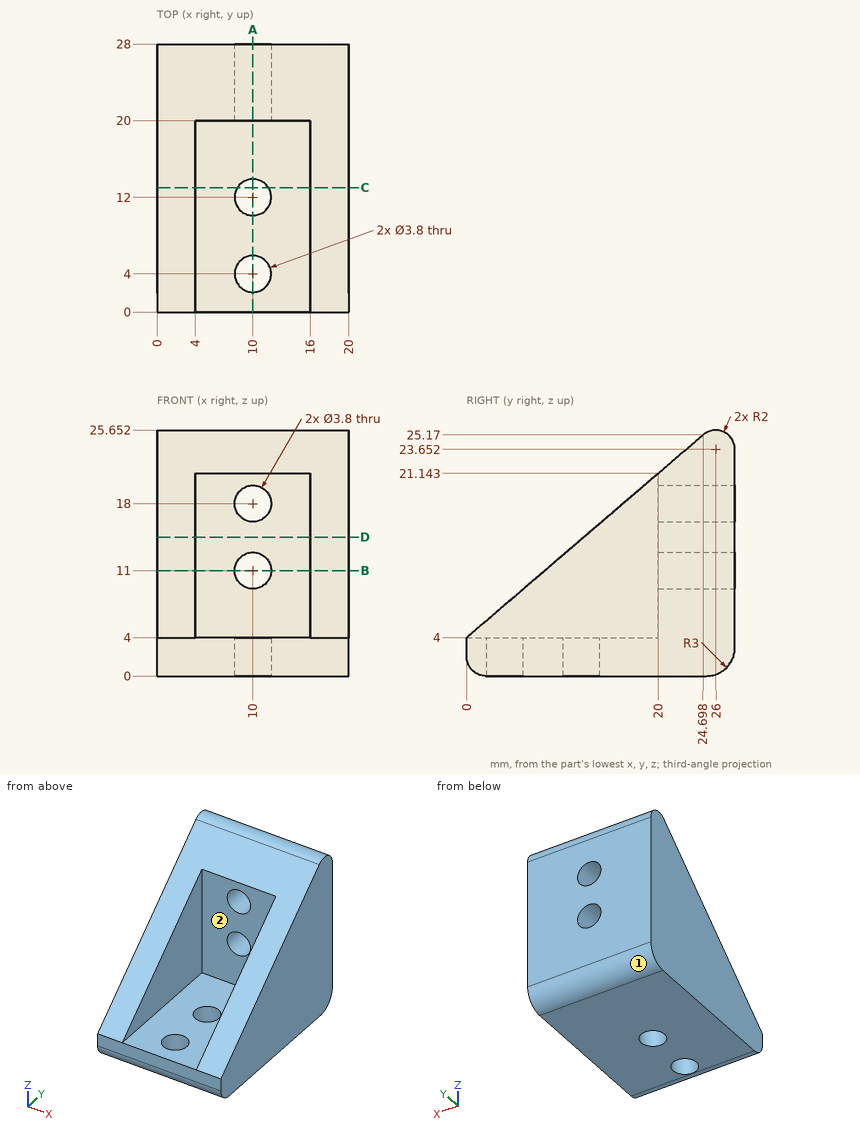
The drawing under review shows one solid part. Ordinate dimensions are in mm from its lowest x, y, z. A direction names the side the tool comes from. Give positions to 0.01 mm unless a question says otherwise; leave off trailing zeros. Order: outer loops, then holes, each group sorted by start corner. A loop starts at its lowest first (then second) coordinate and runs counter-clockwise, first axis right, second up. Notation, with made-up numbers: (71, 73) -> (83, 73) arc R26 ccw to (83, 104) -> close; hole circle Ø10 at (10.25, 65). An arc over 180 degrees is marked (long way). Write item = value, one per line. Start each with the question number.
(1) For pin 1 (1 mm diameter, centred on x = 4, y = 16.5, fed in from +Z); pin 2 (3.5 mm diameter, centred on x = 10, y = 15, fed in from +Z); pin 3 (8 mm diameter, centred on y = 14, z = 7.5, fed in from -X); pin 4 (6 mm diameter, centred on x = 8, z = 15, fed in from -Y), all flat-tipped, find the tip position at first contact; note any pin that passes through.
(2) We need section A-A on x = 10. Write out the cut boundary in (y, z).
(3) We need section C-C on y = 13. Write out the cut boundary in (x, z) (1 decimal), plus the area to 3 significant figures.
(4) For the marked faces 1 and 2, list the 3-axis set-ups (+Z, -Z, +X, -X, +Y, -Y) from which the entire face can be reached by the end or side of a thin tool; tool diameter is ignored.
(5) To check wall thickness, follow line 1 along X through (y, z) = (6, 7.75); line 2 along Y through (x, z) = (10, 1) (1 decimal); line 3 along X through (y, z) = (23.5, 18). State the ranges of each line that lie inside material, in increasing order.
(6) We need section B-B on z = 11. Write out the cut boundary in (x, y), plus the area to 3 significant figures.
(7) We need section D-D on z = 14.5. Write out the cut boundary in (x, y).
Numbers:
q1.pin_1 = 18.57
q1.pin_2 = 4
q1.pin_3 = 0
q1.pin_4 = 20
q2.outline = (0, 2) arc R2 ccw to (2, 0) -> (2.1, 0) -> (2.1, 4) -> (0, 4) -> close; (5.9, 0) -> (10.1, 0) -> (10.1, 4) -> (5.9, 4) -> close; (13.9, 0) -> (25, 0) arc R3 ccw to (28, 3) -> (28, 9.1) -> (20, 9.1) -> (20, 4) -> (13.9, 4) -> close; (20, 12.9) -> (28, 12.9) -> (28, 16.1) -> (20, 16.1) -> close; (20, 19.9) -> (28, 19.9) -> (28, 23.65) arc R2 ccw to (24.7, 25.17) -> (20, 21.14) -> close
q3.outline = (0, 0) -> (8.4, 0) -> (8.4, 4) -> (4, 4) -> (4, 15.1) -> (0, 15.1) -> close; (11.6, 0) -> (20, 0) -> (20, 15.1) -> (16, 15.1) -> (16, 4) -> (11.6, 4) -> close
q3.area = 156 mm^2
q4.face_1 = -Z, +X, -X, +Y
q4.face_2 = +Z, -Y
q5.line_1 = 0 to 4, 16 to 20
q5.line_2 = 0.3 to 2.1, 5.9 to 10.1, 13.9 to 27.2
q5.line_3 = 0 to 8.1, 11.9 to 20
q6.outline = (0, 8.17) -> (4, 8.17) -> (4, 20) -> (8.1, 20) -> (8.1, 28) -> (0, 28) -> close; (11.9, 20) -> (16, 20) -> (16, 8.17) -> (20, 8.17) -> (20, 28) -> (11.9, 28) -> close
q6.area = 224 mm^2
q7.outline = (0, 12.25) -> (4, 12.25) -> (4, 20) -> (16, 20) -> (16, 12.25) -> (20, 12.25) -> (20, 28) -> (0, 28) -> close
